Geometry: final body of the model. Coordinates: model frame, mm. Give positions to 0.01 mm unless a question says otherwise; leave off trailing zeros. Write each loop counter-clockwise with the first axis right and the second up, starting at its lowest first coordinate (ties: lowest second). Pieces come first, ordered by that corner, then holes. Notation, with made-up numbers: M -40,58.5 L -27,58.5 A26 ccw -27,93.5 Z; hole C -19.75,74.25 d5. An arc over 180 degrees is marked long. One line per question, with ' | ' between items.
from build123d import *

# Parameters (mm, degrees)
WYCI_GNI_CIE_CIENKA_CIANKA1_DEPTH      = 400
WYCI_GNI_CIE_CIENKA_CIANKA1_DEPTH_BACK = 400


# Read off the part's stored shape, not the designer's step: Lustro1
with BuildPart() as part:
    # Szkic1 → Wyciągnięcie-cienka ścianka1 (new, two sides: drawn at the far end of the back side and taken through both)
    with BuildSketch(Plane(origin=(0, 0, 0), x_dir=(1, 0, 0), z_dir=(0, 1, 0)).offset(-WYCI_GNI_CIE_CIENKA_CIANKA1_DEPTH_BACK)):
        Polygon((961.046281695, -470.048059203), (543.39, -106.98499256), (517.88, -106.98499256), (517.88, -107.48499256), (543.20305766, -107.48499256), (960.718252181, -470.425413993), align=None)
    extrude(amount=WYCI_GNI_CIE_CIENKA_CIANKA1_DEPTH + WYCI_GNI_CIE_CIENKA_CIANKA1_DEPTH_BACK)

    # Cięcie powierzchnią1
    split(bisect_by=Plane(origin=(-24.349944471, -199.016868, -21.167083796), x_dir=(0.7449832908348125, -0.1600276007809854, 0.6476040946173941), z_dir=(-0.12077436340947467, -0.987112540183885, -0.10498755238005406)), keep=Keep.BOTTOM)

    # Cięcie powierzchnią2
    split(bisect_by=Plane(origin=(110.843151094, -553.888363867, 96.354481224), x_dir=(0.7294998198065532, 0.25630205312360615, 0.6341445185971655), z_dir=(0.19343361492315114, -0.9665967398893007, 0.1681492761005468)), keep=Keep.BOTTOM)

    # Cięcie powierzchnią3
    split(bisect_by=Plane(origin=(-14.708403282, -64.029657214, -16.335336758), x_dir=(0.6328754019353329, -0.32469887066665304, 0.7028793417173329), z_dir=(-0.21726595221314635, -0.9458174471787884, -0.24129828557433775)), keep=Keep.BOTTOM)

    # Lustro1
    split(bisect_by=Plane.ZX, keep=Keep.BOTTOM)

    # Lustro1 2: part across plane


with BuildPart() as part_1:
    add(part.part)
    add(part.part.mirror(Plane.ZX))


solid = part_1.part
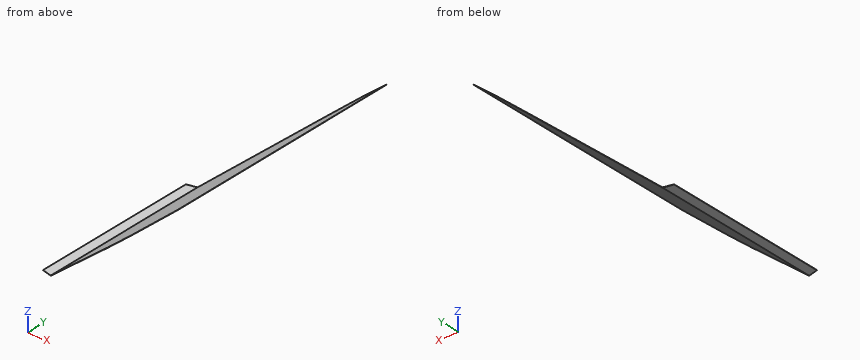
(1) Cut plane C-C, the plane x = 855.5. Return loops of the section in (y, z), then the cut area to 3 significant figures.
Working result:
outline: M -349.22,378.96 L -349.15,378.3 L 349.15,378.3 L 349.22,378.96 Z | area: 463 mm^2
(2) Cut plane B-B, the plane z = 216. Return loops of the section in (x, y).
Working result:
outline: M 668.04,-280.14 L 668.8,-280.31 L 668.8,280.31 L 668.04,280.14 Z
(3) Material intervals for L1, parallel to Z at x = 836, y = 84.5; L2, parallel to Z at x = 885.5, y = -201; L3, parallel to X at y = 4, z = 387, sorted ascending. Write a range as [from, to].
Working result:
L1: z = [361.35, 362.01] | L2: z = [404.38, 405.04] | L3: x = [864.75, 865.51]
(4) First-contact query: P1, Ø3, axis at y = -240.5, z = 377, coming from the -X side; P2, Ø10, axis at x = 707, y = 260, coming from the +Z side; P3, Ø8, axis at x = 607.5, y = -106, coming from the -Z side. Flat tips, straight axial feed; report the tip coordinate or a pass-through.
Working result:
P1: stops at x = 851.52 | P2: stops at z = 254.22 | P3: stops at z = 159.24
(5) Cut plane A-A, the plane y = 11.5. Return loops of the section in (x, z) (3 decimals), then the cut area to 3 significant figures.
Working result:
outline: M 517.88,106.985 L 543.39,106.985 L 961.046,470.048 L 960.718,470.425 L 543.203,107.485 L 517.88,107.485 Z | area: 289 mm^2
